Autodesk Inventor part; units mm, degrees
ref_plane "YZ Plane" through (0, 0, 0) normal (1, 0, 0) x (0, 1, 0)
ref_plane "XZ Plane" through (0, 0, 0) normal (0, 1, 0) x (-1, 0, 0)
ref_plane "XY Plane" through (0, 0, 0) normal (0, 0, 1) x (1, 0, 0)
sketch "Boceto1" plane through (0, 0, 0) normal (0, 0, 1) x (1, 0, 0)
  line L0 (0.25, 8.5) -> (5.35, 8.5)
  line L1 (5.6, 8.25) -> (5.6, 0)
  line L2 (0, 0) -> (0, 8.25)
  line L3 (5.6, 0) -> (5.4774, 0)
  line L4 (0.18, -0.1368) -> (1.78, -0.1368)
  line L5 (2.09, -0.1465) -> (3.59, -0.1465)
  line L6 (3.74, -0.1465) -> (5.24, -0.1465)
  line L7 (0.18, 0) -> (0, 0)
  line L8 (2.09, 0) -> (1.78, 0)
  line L9 (3.59, 0) -> (3.74, 0)
  line L10 (5.24, 0) -> (5.6, 0)
  line L11 (1.1232, 4.6) -> (1.1232, 6.1)
  line L12 (1.1232, 6.1) -> (0, 6.1)
  line L13 (1.1232, 4.6) -> (0, 4.6)
  line L14 (0, 8.25) -> (0, 8.15)
  circle A0 centre (0.35, 8.15) radius 0.15
  circle A1 centre (5.25, 8.15) radius 0.15
  circle A2 centre (0.35, 2.35) radius 0.15
  circle A3 centre (5.25, 2.35) radius 0.15
  arc A4 (0.25, 8.5) -> (0, 8.25) centre (0.25, 8.25) ccw
  arc A5 (5.6, 8.25) -> (5.35, 8.5) centre (5.35, 8.25) ccw
  line L15 (0, 0) -> (5.6, 0)
extrude "Extrusión1" add sketch "Boceto1" against normal blind 0.1
sketch "Boceto2" plane through (0, 0, 0) normal (0, 0, 1) x (1, 0, 0)
  line L0 (0.25, 8.5) -> (5.35, 8.5)
  line L1 (5.6, 8.25) -> (5.6, 0)
  line L2 (0, 0) -> (0, 8.25)
  line L3 (5.6, 0) -> (5.4774, 0)
  line L4 (0.18, -0.1368) -> (1.78, -0.1368)
  line L5 (1.78, -0.1368) -> (1.78, 1.9632)
  line L6 (1.78, 1.9632) -> (0.18, 1.9632)
  line L7 (0.18, 1.9632) -> (0.18, -0.1368)
  line L8 (2.09, -0.1465) -> (3.59, -0.1465)
  line L9 (3.59, -0.1465) -> (3.59, 1.5535)
  line L10 (3.59, 1.5535) -> (2.09, 1.5535)
  line L11 (2.09, 1.5535) -> (2.09, -0.1465)
  line L12 (3.74, -0.1465) -> (5.24, -0.1465)
  line L13 (5.24, -0.1465) -> (5.24, 1.5535)
  line L14 (5.24, 1.5535) -> (3.74, 1.5535)
  line L15 (3.74, 1.5535) -> (3.74, -0.1465)
  line L16 (0.18, 0) -> (0, 0)
  line L17 (2.09, 0) -> (1.78, 0)
  line L18 (3.59, 0) -> (3.74, 0)
  line L19 (5.24, 0) -> (5.6, 0)
  line L20 (1.1232, 4.6) -> (1.1232, 6.1)
  line L21 (1.1232, 6.1) -> (0, 6.1)
  line L22 (1.1232, 4.6) -> (0, 4.6)
  line L23 (0, 8.25) -> (0, 8.15)
  circle A0 centre (0.35, 8.15) radius 0.15
  circle A1 centre (5.25, 8.15) radius 0.15
  circle A2 centre (0.35, 2.35) radius 0.15
  circle A3 centre (5.25, 2.35) radius 0.15
  arc A4 (0.25, 8.5) -> (0, 8.25) centre (0.25, 8.25) ccw
  arc A5 (5.6, 8.25) -> (5.35, 8.5) centre (5.35, 8.25) ccw
extrude "Extrusión2" add sketch "Boceto2" along normal blind 1.9 contours L13 L12 L15 L14 | L7 L6 L5 L4 | L9 L8 L11 L10
sketch "Boceto3" plane through (0, 0, 0) normal (0, 0, 1) x (1, 0, 0)
  line L0 (0.25, 8.5) -> (5.35, 8.5)
  line L1 (5.6, 8.25) -> (5.6, 0)
  line L2 (0, 0) -> (0, 8.25)
  line L3 (5.6, 0) -> (5.4774, 0)
  line L4 (0.18, -0.1368) -> (1.78, -0.1368)
  line L5 (1.78, -0.1368) -> (1.78, 1.9632)
  line L6 (1.78, 1.9632) -> (0.18, 1.9632)
  line L7 (0.18, 1.9632) -> (0.18, -0.1368)
  line L8 (2.09, -0.1465) -> (3.59, -0.1465)
  line L9 (3.59, -0.1465) -> (3.59, 1.5535)
  line L10 (3.59, 1.5535) -> (2.09, 1.5535)
  line L11 (2.09, 1.5535) -> (2.09, -0.1465)
  line L12 (3.74, -0.1465) -> (5.24, -0.1465)
  line L13 (5.24, -0.1465) -> (5.24, 1.5535)
  line L14 (5.24, 1.5535) -> (3.74, 1.5535)
  line L15 (3.74, 1.5535) -> (3.74, -0.1465)
  line L16 (0.18, 0) -> (0, 0)
  line L17 (2.09, 0) -> (1.78, 0)
  line L18 (3.59, 0) -> (3.74, 0)
  line L19 (5.24, 0) -> (5.6, 0)
  line L20 (1.1232, 4.6) -> (1.1232, 6.1)
  line L21 (1.1232, 6.1) -> (0, 6.1)
  line L22 (1.1232, 4.6) -> (0, 4.6)
  line L23 (0, 8.25) -> (0, 8.15)
  circle A0 centre (0.35, 8.15) radius 0.15
  circle A1 centre (5.25, 8.15) radius 0.15
  circle A2 centre (0.35, 2.35) radius 0.15
  circle A3 centre (5.25, 2.35) radius 0.15
  arc A4 (0.25, 8.5) -> (0, 8.25) centre (0.25, 8.25) ccw
  arc A5 (5.6, 8.25) -> (5.35, 8.5) centre (5.35, 8.25) ccw
  point P0 (0, 0)
extrude "Extrusión3" add sketch "Boceto3" along normal blind 0.6 contours L21 L20 L22 L2
properties part number "learnbotOdroid"
Design review of the part built by this model. Coordinates are the model's own, in mm. A direction names the side the tool comes from. Give positions to 0.01 mm unless a question says otherwise; leave off trailing zeros. Order: outer loops, then holes, each group sorted by start corner. A loop starts at its lowest first (then second) coordinate and runs counter-clockwise, first axis right, second up. Notation, with made-up numbers: (16.5, -31) - (24.5, -31) arc R22 ccw to (24.5, -4) - close; hole circle Ø2 at (25.25, 51.25). An arc over 180 degrees is marked (long way). Write item = value, one per line. Start each with the question number.
Q1. We need section B-B on x = 0.35. State the section outline as (y, z) points, plus the area to 3 significant figures.
Q2. We need section A-A on z = 0.3. State the section outline as (x, y) points.
Q3. Tool access review of faces 5 (the face through (3.59, 1, 1)), 6 (the face through (5, 1.554, 1)), 7 (the face through (0.18, 1, 1)): name each direction out of +Z, -Z, +X, -X, +Y, -Y from which nothing blocks a thin tool from reaching the whole face with its end or side.
Q4. To check wall thickness, follow L1, parallel to X at y = 0.75, z = 1.55; L2, parallel to Y at x = 5.25, z = -0.05; L3, parallel to Y at x = 0.5, z = 0.15. State the ranges of each line that lie inside material, in increasing order. Write a range as from..to.
Q5. Clearance check with flat-ended pins moving along their axes: pin 1 Ø0.6 at (y, z) = (1, 1) entering from -X; pin 2 Ø3 at (x, y) = (3.5, 5.5) entering from +Z; pin 3 Ø0.5 at (x, z) = (1, 1) entering from +Y. State where each tip first meets the part, or that it passes through.
Q6. We need section C-C on z = 0.7. State the section outline as (x, y) points.
Q7. Mouldability with a two-part tool opening along Y and no side actions: class faces 1 (the face through (1.78, 1, 1)), 2 (the face through (1, 1.963, 1)), 3 (the face through (4, -0.146, 1)), 4 (the face through (3, 1.554, 1)) as released by +Y, released by -Y, zero draft, split by the parting line, or undercut.
Q8. We need section D-D on y = 8.15. State the section outline as (x, z) points.
Working result:
q1.outline = (-0.14, 0) - (0, 0) - (0, -0.1) - (2.2, -0.1) - (2.2, 0) - (1.96, 0) - (1.96, 1.9) - (-0.14, 1.9) - close; (2.5, -0.1) - (8, -0.1) - (8, 0) - (6.1, 0) - (6.1, 0.6) - (4.6, 0.6) - (4.6, 0) - (2.5, 0) - close; (8.3, -0.1) - (8.5, -0.1) - (8.5, 0) - (8.3, 0) - close
q1.area = 5.68 mm²
q2.outline = (0, 4.6) - (1.12, 4.6) - (1.12, 6.1) - (0, 6.1) - close; (0.18, -0.14) - (1.78, -0.14) - (1.78, 1.96) - (0.18, 1.96) - close; (2.09, -0.15) - (3.59, -0.15) - (3.59, 1.55) - (2.09, 1.55) - close; (3.74, -0.15) - (5.24, -0.15) - (5.24, 1.55) - (3.74, 1.55) - close
q3.face_5 = +Z, +Y, -Y
q3.face_6 = +Z, +X, +Y
q3.face_7 = +Z, -X, -Y
q4.L1 = 0.18..1.78, 2.09..3.59, 3.74..5.24
q4.L2 = 0..2.2, 2.5..8, 8.3..8.5
q4.L3 = -0.14..1.96, 4.6..6.1
q5.pin_1 = 0.18
q5.pin_2 = 0
q5.pin_3 = 1.96
q6.outline = (0.18, -0.14) - (1.78, -0.14) - (1.78, 1.96) - (0.18, 1.96) - close; (2.09, -0.15) - (3.59, -0.15) - (3.59, 1.55) - (2.09, 1.55) - close; (3.74, -0.15) - (5.24, -0.15) - (5.24, 1.55) - (3.74, 1.55) - close
q7.face_1 = zero draft
q7.face_2 = undercut
q7.face_3 = released by -Y
q7.face_4 = released by +Y
q8.outline = (0, -0.1) - (0.2, -0.1) - (0.2, 0) - (0, 0) - close; (0.5, -0.1) - (5.1, -0.1) - (5.1, 0) - (0.5, 0) - close; (5.4, -0.1) - (5.6, -0.1) - (5.6, 0) - (5.4, 0) - close
